Could you check a few things on this model? Use its own coordinates, in mm. A direction names the side the tool comes from. Coordinates: 2 decimals unless noted, no trailing zeros. Write each loop counter-clockwise with the first axis right and the second up, starting at its lowest first coordinate (ties: lowest second). Pieces come first, ordered by that corner, then holes. Notation, with made-up numbers: (86, -13.75) - (91, -13.75) arc R22 ccw to (91, -5.75) - close; hole circle Ø4 at (4, 42). An arc over 180 degrees is marked (long way). Answer as a JSON object with one key per item and string values. Group by question number.
1) If we section it at B-B (z = 7.5): Write out the boundary of the cut face in (x, y), plus the area to 3 significant figures.
2) On a 3-axis mill with a long thin cutter (end or side, diameter ignored), from which of +Z, -Z, +X, -X, +Y, -Y can I reach the whole of each face in a straight line? I mean faces 1 (the flat face through (0, 20, 6)), 2 (the cylindrical face through (11.43, 7.65, 11.4)), 3 (the cylindrical face through (11.43, 7.65, 0.6)). Say none if no direction works.
3) If we section it at C-C (y = 3): Write out the boundary of the cut face in (x, z).
4) If we section it at A-A (y = 27.5): Write out the boundary of the cut face in (x, z).
5) Please list where these lines run through material, in increasing order: line 1 along X through (y, z) = (6.5, 6); line 2 along Y through (x, z) = (16.5, 2.75); line 3 along X through (y, z) = (32, 3.75).
6) If we section it at D-D (z = 1.25): Write out the boundary of the cut face in (x, y), plus the area to 3 significant figures.
7) We'd pull the mould along X, two halves only. Please class faces 4 (the flat face through (12, 7, 6)), 5 (the flat face through (8, 20, 0)), 6 (the cylindrical face through (10.699, 21.643, 5.944)): released by +X, released by -X, zero draft, split by the parting line, or undercut.
8) Will these pins go through, and if not, where does the flat tip stop? pin 1 Ø4 at (y, z) = (31.5, 4) entering from +X; pin 2 Ø4 at (y, z) = (23, 10) entering from +X; pin 3 Ø1 at (x, y) = (21.5, 25.5) entering from -Z; pin 4 Ø1.5 at (x, z) = (19, 7.5) entering from +Y.
```python
from build123d import *

# Parameters (mm, degrees)
F0_R     = 6
F1_DEPTH = 12
F2_R     = 2


with BuildPart() as f1:
    # F0 (on Top) → F1 (new body)
    with BuildSketch(Plane.XY):
        with BuildLine():
            Line((0, 40), (0, 0))
            Line((0, 0), (12, 0))
            Line((12, 0), (12, 15))
            ThreePointArc((12, 15), (24.5, 27.5), (12, 40))
            Line((12, 40), (0, 40))
        make_face()
        with Locations((12, 27.5)):
            Circle(F0_R, mode=Mode.SUBTRACT)
    extrude(amount=F1_DEPTH)

    # F2
    f2_edges = [f1.edges().sort_by_distance(p)[0] for p in [
        (6, 40, 12),
        (0, 20, 12),
        (6, 0, 12),
        (12, 7.5, 12),
        (24.5, 27.5, 12),
        (6, 27.5, 12),
        (6, 40, 0),
        (0, 20, 0),
        (6, 0, 0),
        (12, 7.5, 0),
        (24.5, 27.5, 0),
        (6, 27.5, 0),
        (0, 40, 6),
        (0, 0, 6),
        (12, 0, 6),
        (12, 15, 6),
    ]]
    fillet(f2_edges, radius=F2_R)


solid = f1.part
```
Here are the results:
{
 "1": {"outline": "(0, 2) arc R2 ccw to (2, 0) - (10, 0) arc R2 ccw to (12, 2) - (12, 13.14) arc R2 cw to (13.72, 15.12) arc R12.5 ccw to (12, 40) - (2, 40) arc R2 ccw to (0, 38) - close; hole circle Ø12 at (12, 27.5)", "area": "610 mm²"},
 "2": {"face 1": "+Z, -Z, -X, +Y, -Y", "face 2": "+Z, +X, -Y", "face 3": "-Z, +X, -Y"},
 "3": {"outline": "(0, 2) arc R2 ccw to (2, 0) - (10, 0) arc R2 ccw to (12, 2) - (12, 10) arc R2 ccw to (10, 12) - (2, 12) arc R2 ccw to (0, 10) - close"},
 "4": {"outline": "(0, 2) arc R2 ccw to (2, 0) - (4, 0) arc R2 ccw to (6, 2) - (6, 10) arc R2 ccw to (4, 12) - (2, 12) arc R2 ccw to (0, 10) - close; (18, 2) arc R2 ccw to (20, 0) - (22.5, 0) arc R2 ccw to (24.5, 2) - (24.5, 10) arc R2 ccw to (22.5, 12) - (20, 12) arc R2 ccw to (18, 10) - close"},
 "5": {"line 1": "x = 0 to 12", "line 2": "y = 15.84 to 23.53, 31.47 to 39.16", "line 3": "x = 0 to 8.03, 15.97 to 23.66"},
 "6": {"outline": "(0.15, 2) arc R1.85 ccw to (2, 0.15) - (10, 0.15) arc R1.85 ccw to (11.85, 2) - (11.85, 13.14) arc R2.15 cw to (13.7, 15.26) arc R12.35 ccw to (12, 39.85) - (2, 39.85) arc R1.85 ccw to (0.15, 38) - close; hole circle Ø12.29 at (12, 27.5)", "area": "588 mm²"},
 "7": {"face 4": "released by +X", "face 5": "zero draft", "face 6": "undercut"},
 "8": {"pin 1": "stops at x = 24.34", "pin 2": "stops at x = 24.25", "pin 3": "stops at z = 0", "pin 4": "stops at y = 38.33"}
}
